Input: part model. Units: mm. Frame: model coordinates. Face numbers are marked on the shaded views. A direction names the side the tool comes from. Coordinates: 2 decimals unless noted, no trailing zeros. Order: outer loops, then holes, each group sorted by start corner. A loop starts at its lowest first (then second) coordinate and runs counter-clockwise, first axis right, second up. Notation, with made-up numbers: (73, -34.5) -> (117, -34.5) arc R25 ccw to (117, -19.5) -> close; hole circle Ø8 at (19.25, 57.5). An arc over 180 degrees is marked (long way). Use one line per item in the form item = value. Start each with the question number.
1) Section query D-D on y = -7. Output: boundary loops of the cut face in (x, z) (3 decimals), then the cut area to 3 significant figures.
2) Section query A-A on y = -0.75. Output: boundary loops of the cut face in (x, z) (1 decimal), then the cut area to 3 significant figures.
3) Pin query (flat end, axial travel): pin 1 (6 mm diameter, centred on x = -13, y = -3, fed in from +Z) (3 decimals); pin 2 (9 mm diameter, centred on x = -9, z = 0, fed in from -Y); pin 3 (1 mm diameter, centred on y = -2, z = -6.5, fed in from -X). Return the tip coordinate at first contact, or that it passes through.
4) Section query B-B on x = -2.5. Output: boundary loops of the cut face in (y, z) (3 decimals), then the cut area to 3 significant figures.
5) Access query for the marked faces 5 and 6. Directions: +Z, -Z, +X, -X, +Y, -Y. A direction counts if a zero-diameter tool reaches every point of the face in a straight line with its end or side. Return the directions, or none.
6) Section query C-C on z = 0. Output: boundary loops of the cut face in (x, y), then the cut area to 3 significant figures.
7) Draft query along Z for the marked faces 1, 2, 3 and 4. Return one class per face: pulls with the +Z half, pulls with the -Z half, needs draft (parallel to the pull), parting line crosses it, or undercut.
8) Ray query, line 1 along Z through (x, y) = (-0.85, -7) (3 decimals); line 2 along X through (y, z) = (-1.65, 0); line 3 along X through (y, z) = (-10.5, 2.5). Return the intervals inside material, ascending.
Autodesk Inventor part; units mm, degrees
ref_plane "YZ Plane" through (0, 0, 0) normal (1, 0, 0) x (0, 1, 0)
ref_plane "XZ Plane" through (0, 0, 0) normal (0, 1, 0) x (-1, 0, 0)
ref_plane "XY Plane" through (0, 0, 0) normal (0, 0, 1) x (1, 0, 0)
sketch "Sketch1" plane through (0, 0, 0) normal (0, 0, 1) x (1, 0, 0)
  line L0 (-4, -13) -> (0, -13)
  line L1 (0, -13) -> (0, 0)
  line L2 (0, 0) -> (-15, 0)
  line L3 (-15, 0) -> (-15, -3)
  line L4 (-15, -3) -> (-4, -3)
  line L5 (-4, -3) -> (-4, -13)
  dimension "d0" = 3
  dimension "d1" = 4
  dimension "d2" = 10
  dimension "d3" = 15
extrude "Extrusion1" add sketch "Sketch1" along normal mid plane 19.05
sketch "Sketch2" plane through (-4, -13, 9.525) normal (-1, 0, 0) x (0, 0, 1)
  line L0 (-19.05, 0) -> (0, 0)
  line L1 (0, 10) -> (0, 0)
  line L2 (-19.05, 10) -> (0, 10)
  line L3 (-19.05, 0) -> (-19.05, 10)
  line L4 (-19.05, 0) -> (-19.05, 10)
  line L5 (-19.05, 13) -> (0, 13)
  line L6 (-19.05, 0) -> (0, 0)
  point P0 (-9.525, 13)
  point P1 (-14.525, 6)
  point P2 (-4.525, 6)
  point P3 (-19.05, 5)
  point P4 (-9.525, 13)
  point P5 (-9.525, 0)
  dimension "d6" = 10
  dimension "d31" = 7
  dimension "d32" = 5
hole "Hole1" at (-4, -7, -5) at (-4, -7, 5) direction (1, 0, 0) diameter 3.4 depth 8.7884
sketch "Sketch3" plane through (-15, 0, 9.525) normal (0, 1, 0) x (1, 0, 0)
  line L0 (15, 19.05) -> (15, 0)
  point P0 (15, 9.525)
  point P1 (3, 9.525)
  point P2 (15, 9.525)
  dimension "d15" = 12
hole "Hole2" at (-12, 0, 0) direction (0, -1, 0) diameter 2.459 depth 8.8
chamfer "Chamfer1" distance 10 distance2 8 1 edges at (-15, -1.5, 9.525) measured on face at (-1.3333, -5.3333, 9.525)
chamfer "Chamfer2" distance 10 distance2 8 1 edges at (-15, -1.5, -9.525) measured on face at (-1.3333, -5.3333, -9.525)
fillet "Fillet1" radius 2 4 edges at (-5, -1.5, -9.525) (-15, -1.5, -1.525) (-15, -1.5, 1.525) (-5, -1.5, 9.525)
fillet "Fillet1" radius 5 2 edges at (-2, -13, -9.525) (-2, -13, 9.525)
properties part number "X-Axis_Z_Endstop_Bracket_LM3047" material "ABS Plastic"
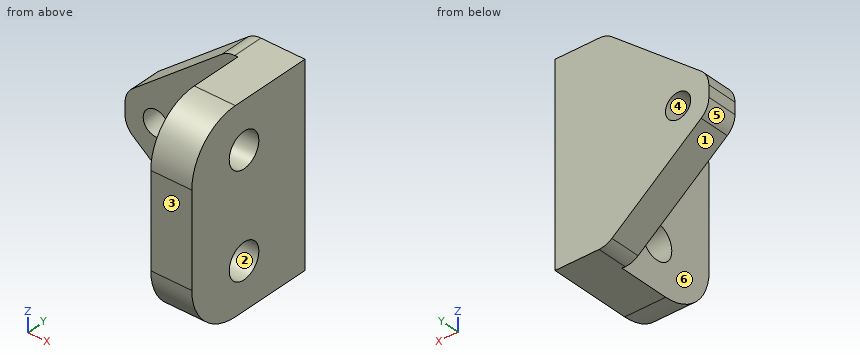
Answers below:
q1.outline = (-4, -9.525) -> (0, -9.525) -> (0, -6.7) -> (-4, -6.7) -> close; (-4, -3.3) -> (0, -3.3) -> (0, 3.3) -> (-4, 3.3) -> close; (-4, 6.7) -> (0, 6.7) -> (0, 9.525) -> (-4, 9.525) -> close
q1.area = 49.0 mm^2
q2.outline = (-15, -0.6) arc R2 ccw to (-14.2, -2.1) -> (-5.5, -9.1) arc R2 ccw to (-4.3, -9.5) -> (0, -9.5) -> (0, 9.5) -> (-4.3, 9.5) arc R2 ccw to (-5.5, 9.1) -> (-14.2, 2.1) arc R2 ccw to (-15, 0.6) -> close; hole circle Ø2.5 at (-12, 0)
q2.area = 201 mm^2
q3.pin_1 = 5.525
q3.pin_2 = -3
q3.pin_3 = -9.41
q4.outline = (-13, -4.525) arc R5 ccw to (-8, -9.525) -> (0, -9.525) -> (0, 9.525) -> (-8, 9.525) arc R5 ccw to (-13, 4.525) -> close; hole circle Ø3.4 at (-7, -5); hole circle Ø3.4 at (-7, 5)
q4.area = 219 mm^2
q5.face_5 = -Z, -X, +Y, -Y
q5.face_6 = +Z, -Z, -X, -Y
q6.outline = (-15, -3) -> (-13.23, -3) -> (-13.23, 0) -> (-15, 0) -> close; (-10.77, -3) -> (-4, -3) -> (-4, -13) -> (0, -13) -> (0, 0) -> (-10.77, 0) -> close
q6.area = 77.6 mm^2
q7.face_1 = pulls with the -Z half
q7.face_2 = undercut
q7.face_3 = needs draft
q7.face_4 = undercut
q8.line_1 = -9.525 to -6.7, -3.3 to 3.3, 6.7 to 9.525
q8.line_2 = -15 to -13.23, -10.77 to 0
q8.line_3 = -4 to 0
